Drawing for the job (mm, zero at the part's lowest x, y, z). A direction names the side the tool comes from. Give positions to 0.01 mm unless a question says otherwise; leave off trailing zeros. Write each loop counter-clockwise with the first axis right and the second up, starting at its lowest first coordinate (ties: lowest second). Pieces come first, ordered by that corner, then holes. Notation, with made-up numbers: M 58.5,44 L 80.5,44 A20 ccw 80.5,83 Z; hole C 34.25,20 d2. An arc over 180 degrees is marked long. Use CSV: the item, a comma, the result in double quotes. Start each with the question number.
1. 3-axis set-ups, long thin cutter, end or side, ignore diameter. For the marked faces 5, 6 and 7: which of +Z, -Z, +X, -X, +Y, -Y reach the whole face in a straight line?
2. Drop flat-ended pins along their axis: pin 1 Ø5.5 at (x, y) = (9, 25) entering from -Z; pin 2 Ø1 at (y, z) = (52.5, 43) entering from -X; pin 3 Ø14 at (y, z) = (42.5, 27.5) entering from +X; pin 4 Ø2 at (x, y) = (61, 69.5) entering from +Z. Give the stop position or say it passes through.
3. Mould opens along X. For the marked faces 1, 2, 3 and 4 say: pulls with the +X half, pulls with the -X half, needs draft (parallel to the pull), parting line crosses it, or undercut.
4. Band-saw the part on C-C, the plane z = 24.5. List the corners of the cut face in (x, y), then the cut area to 3 significant figures.
5. Band-saw the part on B-B, the plane x = 50. List the corners of the cut face in (y, z).
6. Drill centre lines: line 1 along Y through (x, z) = (50, 3.65); line 2 along X through (y, z) = (75, 1); line 3 along X through (y, z) = (54, 50). Where is each one in solid material? Low to high. Write a range as from..to.
7. Band-saw the part on A-A, the plane z = 30. Count the separate pieces of the cut face and the enclosed holes in it, then the cut area to 3 significant figures.
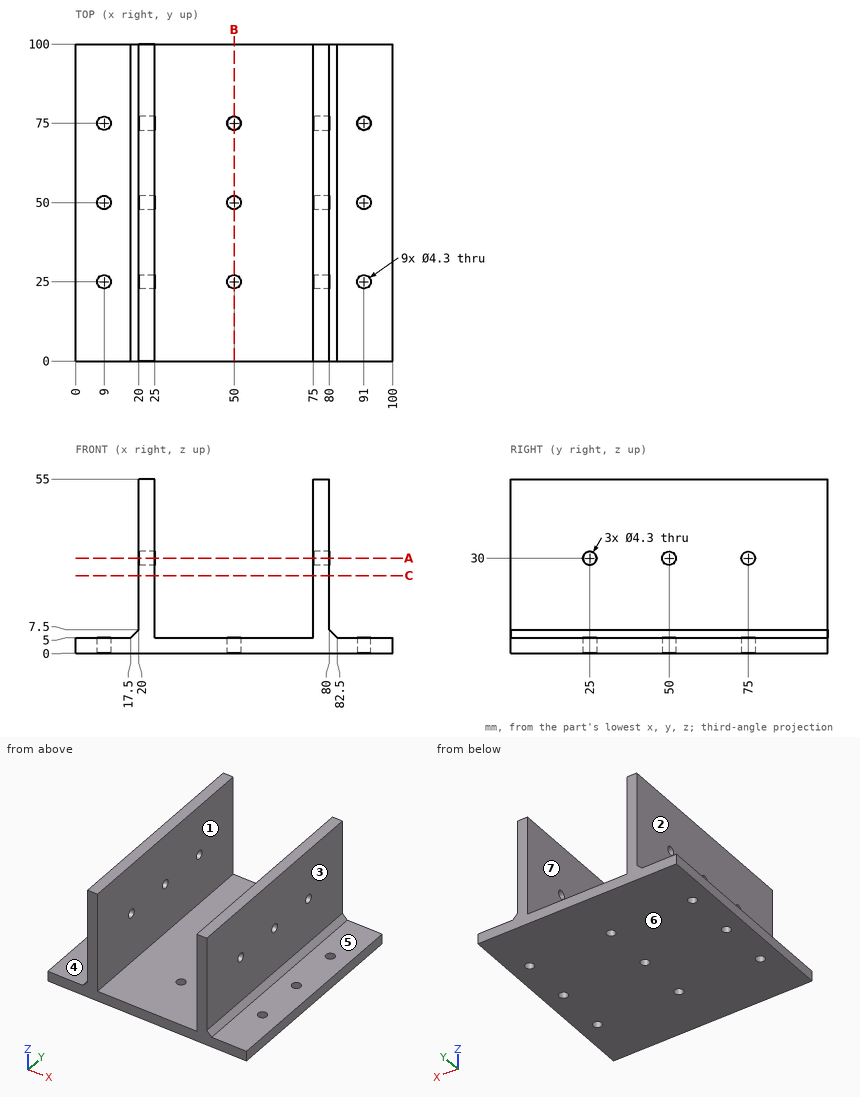
Output:
1,face 5,"+Z, +X, +Y, -Y"
1,face 6,"-Z, +X, -X, +Y, -Y"
1,face 7,"+Z, +Y, -Y"
2,pin 1,"stops at z = 0"
2,pin 2,"stops at x = 20"
2,pin 3,"stops at x = 80"
2,pin 4,"stops at z = 5"
3,face 1,"undercut"
3,face 2,"pulls with the -X half"
3,face 3,"pulls with the +X half"
3,face 4,"needs draft"
4,outline,"M 20,0 L 25,0 L 25,100 L 20,100 Z; M 75,0 L 80,0 L 80,100 L 75,100 Z"
4,area,"1,000 mm²"
5,outline,"M 0,0 L 22.85,0 L 22.85,5 L 0,5 Z; M 27.15,0 L 47.85,0 L 47.85,5 L 27.15,5 Z; M 52.15,0 L 72.85,0 L 72.85,5 L 52.15,5 Z; M 77.15,0 L 100,0 L 100,5 L 77.15,5 Z"
6,line 1,"y = 0..22.85, 27.15..47.85, 52.15..72.85, 77.15..100"
6,line 2,"x = 0..6.85, 11.15..47.85, 52.15..88.85, 93.15..100"
6,line 3,"x = 20..25, 75..80"
7,separate pieces,"8"
7,enclosed holes,"0"
7,area,"871 mm²"
